Source: CAD feature listing. Evaluate the final solid. Frame: model axes, mm. A direction names the side the tool comes from. Give positions to 0.01 mm unless a question says otherwise; leave off trailing zeros. Order: outer loops, then holes, each group sorted by start corner. A loop starts at its lowest first (then second) coordinate and runs counter-clockwise, first axis right, second up.
from build123d import *

# Parameters (mm, degrees)
SKETCH2_W           = 1500
SKETCH2_H           = 1500
BOSS_EXTRUDE1_DEPTH = 10
BOSS_EXTRUDE2_DEPTH = 110


with BuildPart() as part:
    # Sketch2 → Boss-Extrude1 (new body)
    with BuildSketch(Plane(origin=(0, 0, 0), x_dir=(1, 0, 0), z_dir=(0, 1, 0))):
        Rectangle(SKETCH2_W, SKETCH2_H)
    extrude(amount=BOSS_EXTRUDE1_DEPTH)

    # Sketch3 → Boss-Extrude2 (add)
    with BuildSketch(Plane(origin=(0, 10, 0), x_dir=(1, 0, 0), z_dir=(0, 1, 0))):
        with BuildLine():
            ThreePointArc((750, -600), (-204.594154602, -204.594154602), (-600, 750))
            Line((-600, 750), (-620, 750))
            ThreePointArc((-620, 750), (-218.736290226, -218.736290226), (750, -620))
            Line((750, -620), (750, -600))
        make_face()
        with BuildLine():
            Line((620, 750), (600, 750))
            ThreePointArc((600, 750), (643.933982822, 643.933982822), (750, 600))
            Line((750, 600), (750, 620))
            ThreePointArc((750, 620), (658.076118446, 658.076118446), (620, 750))
        make_face()
    extrude(amount=BOSS_EXTRUDE2_DEPTH)


solid = part.part
1) Section query C-C on x = 116. Output: boundary loops of the cut face in (y, z), and give its area (3 significant figures).
Checks:
outline: (0, -750) - (10, -750) - (10, 441.87) - (120, 441.87) - (120, 464.47) - (10, 464.47) - (10, 750) - (0, 750) - close
area: 17,500 mm2
2) Section query B-B on z = -579.5. Output: boundary loops of the cut face in (x, y).
Checks:
outline: (-750, 0) - (750, 0) - (750, 10) - (-589.19, 10) - (-589.19, 120) - (-609.35, 120) - (-609.35, 10) - (-750, 10) - close
3) Pull-direction query (Z, two-part tool) for faces 1 (the face through (216, 10, -234)), 2 (the face through (652, 120, -659)), 3 (the face through (-229.329, 64.23, 208.026)); classes: +Z half, -Z half, draft (parallel to the pull), parting line (faces both ways), or undercut.
Checks:
face 1: undercut
face 2: draft
face 3: +Z half
4) Ray query, L1, parallel to Y at x = -616, z = -91.5; L2, parallel to Z at x = 78.5, y = 112.5; L3, parallel to Z at x = -265, y = 30. Return the intervals inside material, ascending.
Checks:
L1: y = 0 to 10
L2: z = 421.15 to 444.15
L3: z = 140.1 to 170.15
5) Reachability of faces 4 (the face through (642.77, 64.23, -645.11)), 5 (the face through (699, 10, -700)), 6 (the face through (-337, 10, 274)) from +Z, -Z, +X, -X, +Y, -Y: full face, straight path, thin tool, end or side. Return the list, or none.
Checks:
face 4: +Y
face 5: -Z, +X, +Y
face 6: +Z, -X, +Y
6) First-contact query: pin 1 Ø10 at (y, z) = (42.5, -89.5) entering from +X; pin 2 Ø12 at (x, y) = (-512, 64) entering from +Z; pin 3 Ø8 at (x, z) = (-385.5, -295) entering from +Y. Flat tips, straight axial feed; report the tip coordinate or a pass-through.
Checks:
pin 1: stops at x = -424.57
pin 2: stops at z = -202.86
pin 3: stops at y = 10
7) Section query D-D on z = 648. Output: boundary loops of the cut face in (x, y).
Checks:
outline: (-750, 0) - (750, 0) - (750, 10) - (-750, 10) - close
8) Section query A-A on y = 92.5. Output: boundary loops of the cut face in (x, z), and give its area (3 significant figures).
Checks:
outline: (-620, -750) - (-600, -750) arc R1350 cw to (750, 600) - (750, 620) arc R1370 ccw to start; (600, -750) - (620, -750) arc R130 cw to (750, -620) - (750, -600) arc R150 ccw to start
area: 47,100 mm2
